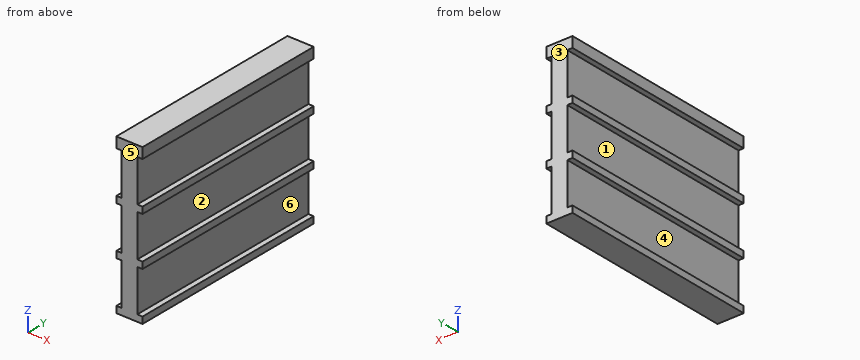
```python
from build123d import *

# Parameters (mm, degrees)
F3_DEPTH = 156


with BuildPart() as f3:
    # F2 (on Front) → F3 (new body)
    with BuildSketch(Plane.XZ):
        Polygon((0, 5), (0, 0), (20, 0), (20, 5), (16, 5), (16, 37), (20, 37), (20, 42), (16, 42), (16, 74), (20, 74), (20, 79), (16, 79), (16, 111), (20, 111), (20, 119), (0, 119), (0, 111), (4, 111), (4, 79), (0, 79), (0, 74), (4, 74), (4, 42), (0, 42), (0, 37), (4, 37), (4, 5), align=None)
    extrude(amount=-F3_DEPTH)


solid = f3.part
```
The listing builds one solid part. Answer for the finished solid, in the listing's coordinates (mm). Face numbers are marked on the shaded views. A direction names the side the tool comes from. Round coordinates to 2 decimals unless told otherwise and drop trailing zeros. Loops run counter-clockwise (first coordinate to the right, second up) from the corner with the lowest first, then second, coordinate; pieces in that order, holes last. Notation, with made-up numbers: (65.25, 9.25) - (121.25, 9.25) arc R33 cw to (121.25, 48.25) - close; hole circle Ø2 at (56.5, 39). An arc over 180 degrees is marked (long way). Return JSON: item names as keys, results as strings. Group by question number.
1. Consider probe 1 along Z at (x, y) = (2.25, 106.5); probe 2 along X at (y, z) = (140, 106.5). Determine where each line is inside the solid, lowest interval first.
2. Which of the six approach directions +Z, -Z, +X, -X, +Y, -Y give full straight-line access (tool end or side, diameter ignored) to the marked faces 4, 5 and 6?
3. The part is cut by section A-A on y = 62. Determine the outline of the cut face in (x, z).
4. The mould has two halves that part along X. Classify the marked faces 1, 2 and 3: pulls with the +X half, pulls with the -X half, needs draft (parallel to the pull), parting line crosses it, or undercut.
5. Each of these flat-tipped pins is pushed along its axis until it touches: P1, Ø16, axis at y = 106.5, z = 92, coming from the +X side; P2, Ø6, axis at y = 28, z = 56, coming from the -X side. Where does it stop, or does it pass through?
6. The part is cut by section B-B on z = 72. Determine the outline of the cut face in (x, y), then the cut area to 3 significant figures.
Resolved:
{
 "1": {"probe 1": "z = 0 to 5, 37 to 42, 74 to 79, 111 to 119", "probe 2": "x = 4 to 16"},
 "2": {"face 4": "-X, +Y, -Y", "face 5": "+Z, -Z, +X, -X, -Y", "face 6": "+X, +Y, -Y"},
 "3": {"outline": "(0, 0) - (20, 0) - (20, 5) - (16, 5) - (16, 37) - (20, 37) - (20, 42) - (16, 42) - (16, 74) - (20, 74) - (20, 79) - (16, 79) - (16, 111) - (20, 111) - (20, 119) - (0, 119) - (0, 111) - (4, 111) - (4, 79) - (0, 79) - (0, 74) - (4, 74) - (4, 42) - (0, 42) - (0, 37) - (4, 37) - (4, 5) - (0, 5) - close"},
 "4": {"face 1": "pulls with the -X half", "face 2": "pulls with the +X half", "face 3": "needs draft"},
 "5": {"P1": "stops at x = 16", "P2": "stops at x = 4"},
 "6": {"outline": "(4, 0) - (16, 0) - (16, 156) - (4, 156) - close", "area": "1,870 mm²"}
}
